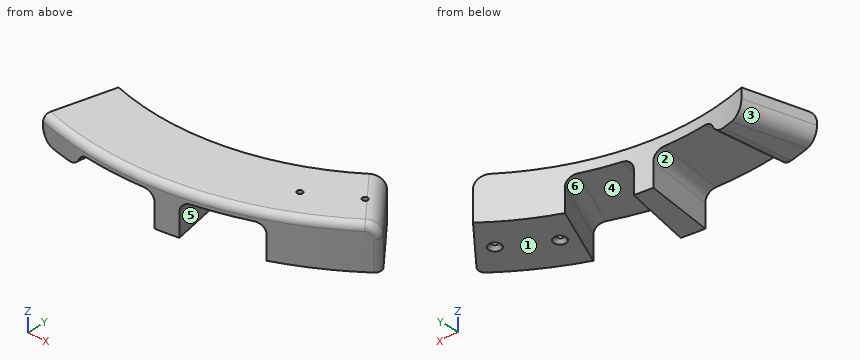
```python
from build123d import *

# Parameters (mm, degrees)
CYLINDER017_R               = 0.8
CYLINDER017_DEPTH           = 20
CYLINDER018_R               = 0.8
CYLINDER018_DEPTH           = 20
CYLINDER019_R               = 0.8
CYLINDER019_DEPTH           = 20
CYLINDER020_R               = 0.8
CYLINDER020_DEPTH           = 20
FUSION007_PLACEMENT_ANGLE   = 10
FUSION008_PLACEMENT_ANGLE   = 297
CYLINDER015_W               = 95
CYLINDER015_H               = 10
CYLINDER015_ANGLE           = 14
CYLINDER015_PLACEMENT_ANGLE = 263
FILLET_R                    = 3
BOX_W                       = 30
BOX_H                       = 30
BOX_DEPTH                   = 8
CYLINDER029_W               = 95
CYLINDER029_H               = 10
CYLINDER029_ANGLE           = 13
CYLINDER029_PLACEMENT_ANGLE = 281
FILLET026_R                 = 3
CYLINDER016_W               = 75
CYLINDER016_H               = 19
CYLINDER016_ANGLE           = 140
CYLINDER016_PLACEMENT_ANGLE = 250
CYLINDER014_W               = 95
CYLINDER014_H               = 13
CYLINDER014_ANGLE           = 55
CYLINDER014_PLACEMENT_ANGLE = 255
FILLET013_R                 = 4
FILLET014_R                 = 2
FILLET027_R                 = 4
CHAMFER_SIZE                = 1


with BuildPart() as cylinder017:
    # Cylinder017 → Cylinder017 (new body)
    with BuildSketch(Plane(origin=(85, 0, 0), x_dir=(1, 0, 0), z_dir=(0, 0, 1))):
        Circle(CYLINDER017_R)
    extrude(amount=CYLINDER017_DEPTH)


with BuildPart() as fusion006:
    # Cylinder018 → Cylinder018 (new body)
    with BuildSketch(Plane(origin=(-85, 0, 0), x_dir=(1, 0, 0), z_dir=(0, 0, 1))):
        Circle(CYLINDER018_R)
    extrude(amount=CYLINDER018_DEPTH)

    # Fusion006: union Cylinder017
    add(cylinder017.part)


with BuildPart() as cylinder019:
    # Cylinder019 → Cylinder019 (new body)
    with BuildSketch(Plane(origin=(85, 0, 0), x_dir=(1, 0, 0), z_dir=(0, 0, 1))):
        Circle(CYLINDER019_R)
    extrude(amount=CYLINDER019_DEPTH)


with BuildPart() as obj1:
    # Cylinder020 → Cylinder020 (new body)
    with BuildSketch(Plane(origin=(-85, 0, 0), x_dir=(1, 0, 0), z_dir=(0, 0, 1))):
        Circle(CYLINDER020_R)
    extrude(amount=CYLINDER020_DEPTH)

    # Fusion007: union Cylinder019
    add(cylinder019.part)


with BuildPart() as obj1_1:
    # Fusion007 placement: moved
    add(obj1.part.rotate(Axis((0, 0, 0), (0, 0, 1)), FUSION007_PLACEMENT_ANGLE))

    # Fusion008: union Fusion006
    add(fusion006.part)


with BuildPart() as obj1_2:
    # Fusion008 placement: moved
    add(obj1_1.part.rotate(Axis((0, 0, 0), (0, 0, 1)), FUSION008_PLACEMENT_ANGLE))


with BuildPart() as fillet_body:
    # Cylinder015 → Cylinder015 (revolve)
    with BuildSketch(Plane.XZ):
        with Locations((47.5, 5)):
            Rectangle(CYLINDER015_W, CYLINDER015_H)
    revolve(axis=Axis((0, 0, 0), (0, 0, 1)), revolution_arc=CYLINDER015_ANGLE)


with BuildPart() as fillet_body_1:
    # Cylinder015 placement: moved
    add(fillet_body.part.moved(Location((0, 0, 2))).rotate(Axis((0, 0, 2), (0, 0, 1)), CYLINDER015_PLACEMENT_ANGLE))

    # Fillet
    fillet_edges = [fillet_body_1.edges().sort_by_distance(p)[0] for p in [
        (5.788794, -47.145942, 12),
        (-5.788794, -47.145942, 12),
    ]]
    fillet(fillet_edges, radius=FILLET_R)


with BuildPart() as cube:
    # Box → Box (new body)
    with BuildSketch(Plane(origin=(-35, -100, 0), x_dir=(1, 0, 0), z_dir=(0, 0, 1))):
        with Locations((15, 15)):
            Rectangle(BOX_W, BOX_H)
    extrude(amount=BOX_DEPTH)


with BuildPart() as fusion:
    # Cylinder029 → Cylinder029 (revolve)
    with BuildSketch(Plane.XZ):
        with Locations((47.5, 5)):
            Rectangle(CYLINDER029_W, CYLINDER029_H)
    revolve(axis=Axis((0, 0, 0), (0, 0, 1)), revolution_arc=CYLINDER029_ANGLE)


with BuildPart() as fusion_1:
    # Cylinder029 placement: moved
    add(fusion.part.moved(Location((0, 0, 2))).rotate(Axis((0, 0, 2), (0, 0, 1)), CYLINDER029_PLACEMENT_ANGLE))

    # Fillet026
    fillet026_edges = [fusion_1.edges().sort_by_distance(p)[0] for p in [
        (19.319991, -43.393409, 12),
        (9.063427, -46.627291, 12),
    ]]
    fillet(fillet026_edges, radius=FILLET026_R)

    # Fusion: union Fillet body, Cube
    add(fillet_body_1.part)
    add(cube.part)


with BuildPart() as cylinder016:
    # Cylinder016 → Cylinder016 (revolve)
    with BuildSketch(Plane.XZ):
        with Locations((37.5, 9.5)):
            Rectangle(CYLINDER016_W, CYLINDER016_H)
    revolve(axis=Axis((0, 0, 0), (0, 0, 1)), revolution_arc=CYLINDER016_ANGLE)


with BuildPart() as cylinder016_1:
    # Cylinder016 placement: moved
    add(cylinder016.part.moved(Location((0, 0, 2))).rotate(Axis((0, 0, 2), (0, 0, 1)), CYLINDER016_PLACEMENT_ANGLE))


with BuildPart() as obj2:
    # Cylinder014 → Cylinder014 (revolve)
    with BuildSketch(Plane.XZ):
        with Locations((47.5, 6.5)):
            Rectangle(CYLINDER014_W, CYLINDER014_H)
    revolve(axis=Axis((0, 0, 0), (0, 0, 1)), revolution_arc=CYLINDER014_ANGLE)


with BuildPart() as obj2_1:
    # Cylinder014 placement: moved
    add(obj2.part.moved(Location((0, 0, 2))).rotate(Axis((0, 0, 2), (0, 0, 1)), CYLINDER014_PLACEMENT_ANGLE))

    # Cut: cut Cylinder016
    add(cylinder016_1.part, mode=Mode.SUBTRACT)

    # Fillet013
    fillet013_edges = [obj2_1.edges().sort_by_distance(p)[0] for p in [
        (54.636947, -65.113778, 15),
    ]]
    fillet(fillet013_edges, radius=FILLET013_R)

    # Fillet014
    fillet014_edges = [obj2_1.edges().sort_by_distance(p)[0] for p in [
        (18.604179, -93.160531, 15),
    ]]
    fillet(fillet014_edges, radius=FILLET014_R)

    # Cut018: cut Fusion
    add(fusion_1.part, mode=Mode.SUBTRACT)

    # Fillet027
    fillet027_edges = [obj2_1.edges().sort_by_distance(p)[0] for p in [
        (-10.358894, -84.366423, 8),
        (-21.999619, -82.103695, 8),
    ]]
    fillet(fillet027_edges, radius=FILLET027_R)

    # Cut019: cut obj1
    add(obj1_2.part, mode=Mode.SUBTRACT)

    # Chamfer
    chamfer_edges = [obj2_1.edges().sort_by_distance(p)[0] for p in [
        (38.226, -75.022749, 2),
        (50.672825, -67.24511, 2),
    ]]
    chamfer(chamfer_edges, length=CHAMFER_SIZE)


solid = obj2_1.part
```
Can you work these out from the model? Positions are in its coordinate system, mm. Face numbers are marked on the shaded views. A direction names the side the tool comes from. Give positions to 0.01 mm unless a question says otherwise; leave off trailing zeros. Write each loop counter-clockwise with the first axis right and the second up, starting at its lowest first coordinate (ties: lowest second). Pieces come first, ordered by that corner, then holes. Notation, with made-up numbers: (-2, 20) -> (51, 20) arc R20 ccw to (51, 33) -> close; hole circle Ø8 at (-15, 64). An arc over 180 degrees is marked (long way). One line per item, written item: value.
Q1. We'd pull the mould along Y, two halves only. Please class the marked faces 1, 2 and 3: +Y half, -Y half, draft (parallel to the pull), parting line (faces both ways), or undercut.
Results found:
face 1: draft
face 2: -Y half
face 3: +Y half
Q2. For P1, Ø1.4, axis at x = 51.15, y = -67.88, coming from the +Z side; P2, Ø6.5, axis at x = -17, y = -80, coming from the -Z side; P3, Ø3, axis at y = -62, z = 13.5, coming from the -X side; P4, Ø6, axis at x = 26, y = -81, coming from the -Z side, each with a flat end and sliding along its axis, tell me the tip position at first contact or that it passes through.
Results found:
P1: passes through
P2: stops at z = 8
P3: stops at x = 39.91
P4: stops at z = 12
Q3. Which directions (+Z, -Z, +X, -X, +Y, -Y) give clear straight access to the entire face, cutting with the end or side of a thin tool? Please do the marked faces 4, 5 and 6.
Results found:
face 4: -Z
face 5: -Z, +Y
face 6: -Z, -Y
Q4. Please list where these lines run through material, in increasing order: line 1 (Z direction, x = 6, y = -88.5); line 2 (X direction, y = -76, z = 5.75); line 3 (X direction, y = -91.5, z = 10). Write a range as [from, to].
Results found:
line 1: z = [12, 15]
line 2: x = [9.33, 14.77], [33.84, 37.83], [39.34, 57]
line 3: x = [-23.96, -11.09], [11.06, 17.96]
Q5. Imagine slicing it at A-A on z = 5. Please give me the cut outline in (x, y), and give its area (3 significant figures).
Results found:
outline: (9.14, -74.44) -> (11.58, -94.29) arc R95 ccw to (18.13, -93.25) -> (14.31, -73.62) arc R75 cw to start; (30.51, -68.52) -> (38.64, -86.79) arc R95 ccw to (59.49, -74.07) arc R2 ccw to (59.77, -71.23) -> (48.21, -57.45) arc R75 cw to start; hole circle Ø1.6 at (38.59, -75.74); hole circle Ø1.6 at (51.15, -67.88)
area: 589 mm^2
